Can you work these out from the model? Positions are in its coordinate system, mm. Face numbers are marked on the shaded views. A direction names the side the tool comes from. Round coordinates to 2 decimals unless told otherwise and drop trailing zeros. Order: outer loops, then holes, each group sorted by start corner. A loop starts at its lowest first (then second) coordinate and runs counter-clockwise, first axis right, second up.
Q1. We'd pull the mould along X, two halves only. Please class the marked faces 4, 5, 6 and 7: pulls with the +X half, pulls with the -X half, needs draft (parallel to the pull), parting line crosses it, or undercut.
Q2. If I drill on line 1 (Y direction, x = 2.5, z = 3); line 2 (Y direction, x = 3.25, z = -5.5); line 3 (X direction, y = 17.5, z = 0.25), over which ranges is the centre line in solid material (lowest first)?
Q3. If we section it at C-C (x = -2.75): Please give me the cut outline in (y, z).
Q4. If we section it at B-B (y = 44): Please give me the cut outline in (x, z).
Q5. If we section it at A-A (z = 0): Please give me the cut outline in (x, y).
Q6. For the marked faces 1, 2 and 3, which set-ups out of +Z, -Z, +X, -X, +Y, -Y let a thin tool reach every point of the face, with its end or its side?
Q7. Will these pins go through, and if not, where does the flat tip stop? P1, Ø8, axis at x = -3, y = 48, coming from the -Z side; P2, Ø6, axis at x = 0, y = 29.5, coming from the -Z side; P3, Ø2, axis at y = 25, z = -3.5, coming from the +X side.
Q8. If we section it at D-D (z = -3.5): Please give me the cut outline in (x, y), plus the area to 3 significant figures.
from build123d import *

# Parameters (mm, degrees)
SKETCH1_R           = 5
BOSS_EXTRUDE1_DEPTH = 60
SKETCH2_W           = 3
SKETCH2_H           = 10
CUT_EXTRUDE2_DEPTH  = 30
SKETCH3_R           = 5
CUT_EXTRUDE3_DEPTH  = 15
BOSS_EXTRUDE2_START = -26
SKETCH4_R           = 7
BOSS_EXTRUDE2_DEPTH = 2


with BuildPart() as part:
    # Sketch1 → Boss-Extrude1 (new body)
    with BuildSketch(Plane(origin=(0, 0, 0), x_dir=(1, 0, 0), z_dir=(0, 1, 0))):
        with Locations(Location((1.609928916, 0, 0), (0, 0, 270))):
            Circle(SKETCH1_R)
    extrude(amount=BOSS_EXTRUDE1_DEPTH)

    # Sketch2 → Cut-Extrude2 (cut, symmetric)
    with BuildSketch(Plane.XY):
        with Locations((1.609928916, 46)):
            Rectangle(SKETCH2_W, SKETCH2_H)
    extrude(amount=CUT_EXTRUDE2_DEPTH, both=True, mode=Mode.SUBTRACT)

    # Sketch3 → Cut-Extrude3 (cut)
    with BuildSketch(Plane.XZ):
        with Locations(Location((1.609928916, 0, 0), (0, 0, 270))):
            Circle(SKETCH3_R)
    extrude(amount=-CUT_EXTRUDE3_DEPTH, mode=Mode.SUBTRACT)

    # Sketch4 → Boss-Extrude2 (add)
    with BuildSketch(Plane.XZ.offset(-15).offset(BOSS_EXTRUDE2_START)):
        with Locations(Location((1.609928916, 0, 0), (0, 0, 270))):
            Circle(SKETCH4_R)
    extrude(amount=BOSS_EXTRUDE2_DEPTH)


solid = part.part
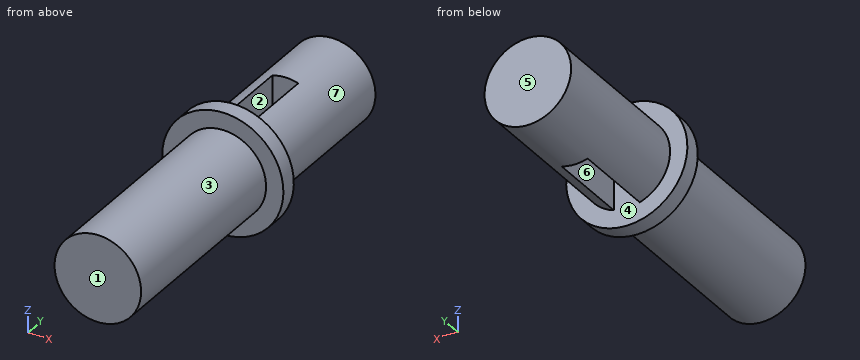
Solution:
1. face 4: undercut
1. face 5: needs draft
1. face 6: undercut
1. face 7: parting line crosses it
2. line 1: y = 15 to 41, 51 to 60
2. line 2: y = 39 to 41
2. line 3: x = -3.38 to 6.6
3. outline: (15, -2.45) - (39, -2.45) - (39, -5.48) - (41, -5.48) - (41, -2.45) - (60, -2.45) - (60, 2.45) - (41, 2.45) - (41, 5.48) - (39, 5.48) - (39, 2.45) - (15, 2.45) - close
4. outline: (0.11, -4.77) - (0.11, 4.77) arc R5 ccw to start; (3.11, -4.77) arc R5 ccw to (3.11, 4.77) - close
5. outline: (-5.39, 39) - (-3.39, 39) - (-3.39, 15) - (6.61, 15) - (6.61, 39) - (8.61, 39) - (8.61, 41) - (6.61, 41) - (6.61, 60) - (-3.39, 60) - (-3.39, 41) - (-5.39, 41) - close; hole (0.11, 41) - (3.11, 41) - (3.11, 51) - (0.11, 51) - close
6. face 1: +Z, -Z, +X, -X, -Y
6. face 2: +Z, -Z
6. face 3: -Y
7. P1: stops at z = -4.77
7. P2: stops at z = -5
7. P3: stops at x = 5.94
8. outline: (-4.45, 39) - (-1.96, 39) - (-1.96, 15) - (5.18, 15) - (5.18, 39) - (7.67, 39) - (7.67, 41) - (5.18, 41) - (5.18, 60) - (-1.96, 60) - (-1.96, 41) - (-4.45, 41) - close; hole (0.11, 41) - (3.11, 41) - (3.11, 51) - (0.11, 51) - close
8. area: 301 mm2
